Input: part model. Units: mm. Frame: model coordinates. Face numbers are marked on the shaded views. Coordinates: 2 decimals unless noted, no trailing zeros. Loops run counter-clockwise (first coordinate to the right, second up) from the corner with the lowest first, then second, coordinate; pieces in that order, holes last. Notation, with made-up numbers: (-5, 16.5) - (17, 16.5) arc R18 ccw to (17, 40.5) - close; hole circle Ø1 at (5, 29). An arc over 180 degrees is marked (long way). Use a Markdown table: item, result. Add a question column.
1. Section query A-A on z = -1. Return the cut outline in (x, y).
2. Section query B-B on x = 9.65. Return the cut outline in (y, z).
3. Section query C-C on y = 1.85. Return the cut outline in (x, z).
4. Ray query, L1, parallel to X at y = 3.75, z = -1; L2, parallel to X at y = 4.85, z = -1.5; L3, parallel to Z at x = 9.65, y = 1.55. Return the intervals inside material, ascending. Write a range as [from, to].
5. Section query D-D on z = 1.5. Return the cut outline in (x, y), then the cut area to 3 significant figures.
6. Draft query along Z for the marked faces 1, 2 and 3. Return one class per face: released by +Z, released by -Z, zero draft, split by the parting line, or undercut.
7. Contact query for flat-ended pins moving along their axis: P1, Ø1.5, axis at x = 9.5, y = 2.5, coming from the +Z side; P2, Ø2, axis at x = 4, y = 4.5, coming from the -Z side; P3, Ø1, axis at x = 1.5, z = 1.5, coming from the +Y side. Output: stop coordinate, or through.
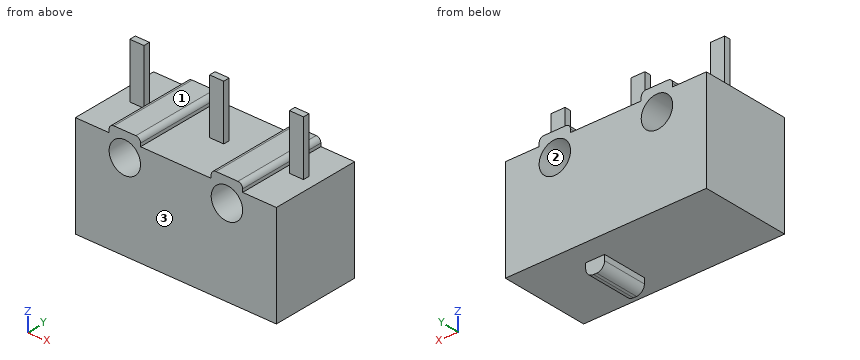
```python
from build123d import *

# Parameters (mm, degrees)
SKETCH1_R           = 1
BOSS_EXTRUDE1_DEPTH = 5.7
SKETCH2_W           = 1.2
SKETCH2_H           = 2.9
BOSS_EXTRUDE2_DEPTH = 0.85
FILLET1_R           = 0.5
SKETCH3_W           = 0.9
SKETCH3_H           = 0.4
BOSS_EXTRUDE3_DEPTH = 3.5


with BuildPart() as part:
    # Sketch1 → Boss-Extrude1 (new body)
    with BuildSketch(Plane(origin=(0, 0, 0), x_dir=(1, 0, 0), z_dir=(0, 1, 0))):
        with BuildLine():
            Line((0, 0), (2.15, 0))
            Line((2.15, 0), (2.15, -0.2))
            ThreePointArc((2.15, -0.2), (2.237867966, -0.412132034), (2.45, -0.5))
            Line((2.45, -0.5), (3.85, -0.5))
            ThreePointArc((3.85, -0.5), (4.062132034, -0.412132034), (4.15, -0.2))
            Line((4.15, -0.2), (4.15, 0))
            Line((4.15, 0), (8.65, 0))
            Line((8.65, 0), (8.65, -0.2))
            ThreePointArc((8.65, -0.2), (8.737867966, -0.412132034), (8.95, -0.5))
            Line((8.95, -0.5), (10.35, -0.5))
            ThreePointArc((10.35, -0.5), (10.562132034, -0.412132034), (10.65, -0.2))
            Line((10.65, -0.2), (10.65, 0))
            Line((10.65, 0), (12.8, 0))
            Line((12.8, 0), (12.8, 6.5))
            Line((12.8, 6.5), (0, 6.5))
            Line((0, 6.5), (0, 0))
        make_face()
        with Locations((3.15, 1)):
            Circle(SKETCH1_R, mode=Mode.SUBTRACT)
        with Locations((9.65, 1)):
            Circle(SKETCH1_R, mode=Mode.SUBTRACT)
    extrude(amount=BOSS_EXTRUDE1_DEPTH)

    # Sketch2 → Boss-Extrude2 (add)
    with BuildSketch(Plane(origin=(0, 0, -6.5), x_dir=(-1, 0, 0), z_dir=(0, 0, -1))):
        with Locations((-8.35, 2.8)):
            Rectangle(SKETCH2_W, SKETCH2_H)
    extrude(amount=BOSS_EXTRUDE2_DEPTH)

    # Fillet1
    fillet1_edges = [part.edges().sort_by_distance(p)[0] for p in [
        (8.95, 2.8, -7.35),
        (7.75, 2.8, -7.35),
    ]]
    fillet(fillet1_edges, radius=FILLET1_R)

    # Sketch3 → Boss-Extrude3 (add)
    with BuildSketch(Plane.XY):
        with Locations((1.45, 3.022147262)):
            Rectangle(SKETCH3_W, SKETCH3_H)
        with Locations((6.53, 3.022147262)):
            Rectangle(SKETCH3_W, SKETCH3_H)
        with Locations((11.61, 3.022147262)):
            Rectangle(SKETCH3_W, SKETCH3_H)
    extrude(amount=BOSS_EXTRUDE3_DEPTH)


solid = part.part
```
Resolved:
| question | item | result |
|---|---|---|
| 1 | outline | (0, 0) - (2.15, 0) - (2.15, 5.7) - (0, 5.7) - close; (4.15, 0) - (8.65, 0) - (8.65, 5.7) - (4.15, 5.7) - close; (10.65, 0) - (12.8, 0) - (12.8, 5.7) - (10.65, 5.7) - close |
| 2 | outline | (0, -6.5) - (5.7, -6.5) - (5.7, -2) - (0, -2) - close; (0, 0) - (5.7, 0) - (5.7, 0.5) - (0, 0.5) - close |
| 3 | outline | (0, -6.5) - (7.75, -6.5) - (7.75, -6.85) arc R0.5 ccw to (8.25, -7.35) - (8.45, -7.35) arc R0.5 ccw to (8.95, -6.85) - (8.95, -6.5) - (12.8, -6.5) - (12.8, 0) - (10.65, 0) - (10.65, 0.2) arc R0.3 ccw to (10.35, 0.5) - (8.95, 0.5) arc R0.3 ccw to (8.65, 0.2) - (8.65, 0) - (4.15, 0) - (4.15, 0.2) arc R0.3 ccw to (3.85, 0.5) - (2.45, 0.5) arc R0.3 ccw to (2.15, 0.2) - (2.15, 0) - (0, 0) - close; hole circle Ø2 at (3.15, -1); hole circle Ø2 at (9.65, -1) |
| 4 | L1 | [0, 2.15], [4.15, 8.65], [10.65, 12.8] |
| 4 | L2 | [0, 2.28], [4.02, 8.78], [10.52, 12.8] |
| 4 | L3 | [-6.5, -2], [0, 0.5] |
| 5 | outline | (1, 2.82) - (1.9, 2.82) - (1.9, 3.22) - (1, 3.22) - close; (6.08, 2.82) - (6.98, 2.82) - (6.98, 3.22) - (6.08, 3.22) - close; (11.16, 2.82) - (12.06, 2.82) - (12.06, 3.22) - (11.16, 3.22) - close |
| 5 | area | 1.08 mm² |
| 6 | face 1 | released by +Z |
| 6 | face 2 | undercut |
| 6 | face 3 | zero draft |
| 7 | P1 | z = 0.5 |
| 7 | P2 | z = -6.5 |
| 7 | P3 | y = 3.22 |
